Source: CAD feature listing. Evaluate the final solid. Frame: model axes, mm. Face numbers are marked on the shaded views. A direction names the side the tool comes from. Round coordinates to 2 decimals unless told otherwise and drop trailing zeros. Order: outer loops, then holes, each group sorted by start corner. A loop starts at its lowest first (then second) coordinate and runs counter-clockwise, first axis right, second up. Notation, with made-up numbers: (66.25, 71.5) - (99.25, 71.5) arc R29 ccw to (99.25, 101.5) - close; hole circle Ø10 at (-29, -4). An arc over 180 degrees is marked (long way). Return JSON: item names as keys, results as strings. Group by question number.
1) Section A-A, the plane y = 116.5. Give the number of separate pieces and of enclosed holes in the cut face, plus the area to 3 significant figures.
2) Ray query, line 1 (Y direction, x = 128.5, z = -52); line 2 (X direction, y = 83, z = 0); line 3 (Z direction, x = -60, y = 99). Return the intervals inside material, ascending. Write a range as from..to.
3) Section D-D, the plane y = 94. Return loops of the section in (x, z).
4) Section C-C, the plane z = 114.5. Return loops of the section in (x, y).
5) Contact query for flat-ended pins moving along their axis: P1, Ø5.5, axis at x = 30.05, z = -30.05, coming from the +Y side; P2, Ø16, axis at x = -55.5, z = -55.5, coming from the +Y side; P3, Ø5, axis at y = 97.5, z = -16.5, coming from the +X side. Output: stop coordinate, or through.
6) Mould query, pull axis X, two halves, no side actions, for the marked faces 3, 4 and 5. Classes: pulls with the +X half, pulls with the -X half, needs draft (parallel to the pull), parting line crosses it, or undercut.
7) Access query for the marked faces 1 and 2. Directions: +Z, -Z, +X, -X, +Y, -Y. A direction counts if a zero-diameter tool reaches every point of the face in a straight line with its end or side. Return the directions, or none.
8) Section B-B, the plane x = 131. Return loops of the section in (y, z), plus the area to 3 significant figures.
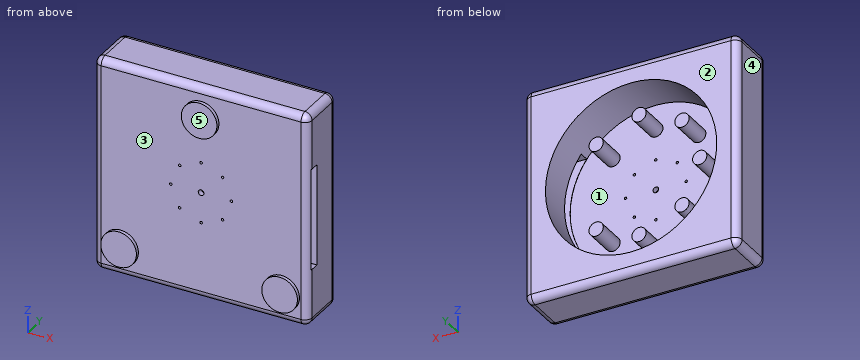
```python
from build123d import *

# Parameters (mm, degrees)
SKETCH_1_W          = 300
SKETCH_1_H          = 300
EXTRUDE_1_DEPTH     = 150
SKETCH_2_R          = 120
CUT_EXTRUDE_1_DEPTH = 62.3
SKETCH_3_R          = 1.75
SKETCH_3_R_2        = 4
CUT_EXTRUDE_2_DEPTH = 10
SKETCH_6_W          = 142.15649329
SKETCH_6_H          = 14
CUT_EXTRUDE_4_DEPTH = 75
SKETCH_11_R         = 10
EXTRUDE_4_DEPTH     = 42.3
FILLET_1_R          = 10
SKETCH_13_W         = 300
SKETCH_13_H         = 300
CUT_EXTRUDE_5_DEPTH = 80
SKETCH_14_R         = 25
EXTRUDE_5_DEPTH     = 5
FILLET_2_R          = 10


with BuildPart() as part:
    # 草图1 → 凸台-拉伸1 (new body)
    with BuildSketch(Plane(origin=(0, 0, 0), x_dir=(1, 0, 0), z_dir=(0, 1, 0))):
        Rectangle(SKETCH_1_W, SKETCH_1_H)
    extrude(amount=EXTRUDE_1_DEPTH)

    # 草图2 → 切除-拉伸1 (cut)
    with BuildSketch(Plane(origin=(0, 150, 0), x_dir=(1, 0, 0), z_dir=(0, 1, 0))):
        with Locations(Location((0, 0, 0), (0, 0, 270))):
            Circle(SKETCH_2_R)
    extrude(amount=-CUT_EXTRUDE_1_DEPTH, mode=Mode.SUBTRACT)

    # 草图3 → 切除-拉伸2 (cut)
    with BuildSketch(Plane(origin=(0, 87.7, 0), x_dir=(1, 0, 0), z_dir=(0, 1, 0))):
        with Locations(Location((42.5, 0, 0), (0, 0, 270))):
            Circle(SKETCH_3_R)
        with Locations(Location((30.0520382, -30.0520382, 0), (0, 0, 270))):
            Circle(SKETCH_3_R)
        with Locations(Location((0, -42.5, 0), (0, 0, 270))):
            Circle(SKETCH_3_R)
        with Locations(Location((-30.0520382, -30.0520382, 0), (0, 0, 270))):
            Circle(SKETCH_3_R)
        with Locations(Location((-42.5, 0, 0), (0, 0, 270))):
            Circle(SKETCH_3_R)
        with Locations(Location((-30.0520382, 30.0520382, 0), (0, 0, 270))):
            Circle(SKETCH_3_R)
        with Locations(Location((0, 42.5, 0), (0, 0, 270))):
            Circle(SKETCH_3_R)
        with Locations(Location((30.0520382, 30.0520382, 0), (0, 0, 270))):
            Circle(SKETCH_3_R)
        with Locations(Location((0, 0, 0), (0, 0, 270))):
            Circle(SKETCH_3_R_2)
    extrude(amount=-CUT_EXTRUDE_2_DEPTH, mode=Mode.SUBTRACT)

    # 草图6 → 切除-拉伸4 (cut)
    with BuildSketch(Plane(origin=(150, 0, 0), x_dir=(0, 0, -1), z_dir=(1, 0, 0))):
        with Locations((0, 95)):
            Rectangle(SKETCH_6_W, SKETCH_6_H)
    extrude(amount=-CUT_EXTRUDE_4_DEPTH, mode=Mode.SUBTRACT)

    # 草图11 → 凸台-拉伸4 (add)
    with BuildSketch(Plane(origin=(0, 87.7, 0), x_dir=(1, 0, 0), z_dir=(0, 1, 0))):
        with Locations(Location((-85, 0, 0), (0, 0, 270))):
            Circle(SKETCH_11_R)
        with Locations(Location((-60.104076401, 60.104076401, 0), (0, 0, 270))):
            Circle(SKETCH_11_R)
        with Locations(Location((0, 85, 0), (0, 0, 270))):
            Circle(SKETCH_11_R)
        with Locations(Location((60.104076401, 60.104076401, 0), (0, 0, 270))):
            Circle(SKETCH_11_R)
        with Locations(Location((60.104076401, -60.104076401, 0), (0, 0, 270))):
            Circle(SKETCH_11_R)
        with Locations(Location((0, -85, 0), (0, 0, 270))):
            Circle(SKETCH_11_R)
        with Locations(Location((-60.104076401, -60.104076401, 0), (0, 0, 270))):
            Circle(SKETCH_11_R)
    extrude(amount=EXTRUDE_4_DEPTH)

    # 圆角1
    fillet_1_edges = [part.edges().sort_by_distance(p)[0] for p in [
        (-150, 150, 0),
        (0, 150, 150),
        (150, 150, 0),
        (0, 0, 150),
        (-150, 0, 0),
        (0, 0, -150),
        (150, 0, 0),
        (150, 75, 150),
        (-150, 75, 150),
        (-150, 75, -150),
        (150, 75, -150),
        (0, 150, -150),
    ]]
    fillet(fillet_1_edges, radius=FILLET_1_R)

    # 草图13 → 切除-拉伸5 (cut)
    with BuildSketch(Plane.XZ):
        Rectangle(SKETCH_13_W, SKETCH_13_H)
    extrude(amount=-CUT_EXTRUDE_5_DEPTH, mode=Mode.SUBTRACT)

    # 草图14 → 凸台-拉伸5 (add)
    with BuildSketch(Plane.XZ.offset(-80)):
        with Locations(Location((0, 104.563725125, 0), (0, 0, 270))):
            Circle(SKETCH_14_R)
        with Locations(Location((-112.815196319, -110.245065947, 0), (0, 0, 270))):
            Circle(SKETCH_14_R)
        with Locations(Location((112.815196319, -110.245065947, 0), (0, 0, 90))):
            Circle(SKETCH_14_R)
    extrude(amount=EXTRUDE_5_DEPTH)

    # 圆角2
    # the kernel refuses this fillet: 10 mm, written as the material it takes off along each edge
    with BuildSketch(Plane(origin=(140, 80, 140), x_dir=(0, 0, 1), z_dir=(-1, 0, 0))) as fillet_2_piece_1:
        with BuildLine():
            CenterArc((10 - FILLET_2_R, FILLET_2_R), FILLET_2_R, 270, 90)
            Line((10, FILLET_2_R), (10, 0))
            Line((10, 0), (10 - FILLET_2_R, 0))
        make_face()
    revolve(axis=Axis((140, 80, 140), (0, 1, 0)), revolution_arc=90, mode=Mode.SUBTRACT)
    with BuildSketch(Plane(origin=(140, 80, -140), x_dir=(1, 0, 0), z_dir=(0, 0, 1))) as fillet_2_piece_2:
        with BuildLine():
            CenterArc((10 - FILLET_2_R, FILLET_2_R), FILLET_2_R, 270, 90)
            Line((10, FILLET_2_R), (10, 0))
            Line((10, 0), (10 - FILLET_2_R, 0))
        make_face()
    revolve(axis=Axis((140, 80, -140), (0, 1, 0)), revolution_arc=90, mode=Mode.SUBTRACT)
    with BuildSketch(Plane(origin=(-140, 80, -140), x_dir=(0, 0, -1), z_dir=(1, 0, 0))) as fillet_2_piece_3:
        with BuildLine():
            CenterArc((10 - FILLET_2_R, FILLET_2_R), FILLET_2_R, 270, 90)
            Line((10, FILLET_2_R), (10, 0))
            Line((10, 0), (10 - FILLET_2_R, 0))
        make_face()
    revolve(axis=Axis((-140, 80, -140), (0, 1, 0)), revolution_arc=90, mode=Mode.SUBTRACT)
    with BuildSketch(Plane(origin=(-140, 80, 140), x_dir=(-1, 0, 0), z_dir=(0, 0, -1))) as fillet_2_piece_4:
        with BuildLine():
            CenterArc((10 - FILLET_2_R, FILLET_2_R), FILLET_2_R, 270, 90)
            Line((10, FILLET_2_R), (10, 0))
            Line((10, 0), (10 - FILLET_2_R, 0))
        make_face()
    revolve(axis=Axis((-140, 80, 140), (0, 1, 0)), revolution_arc=90, mode=Mode.SUBTRACT)
    with BuildSketch(Plane(origin=(-150, 80, -140), x_dir=(1, 0, 0), z_dir=(0, 0, 1)), Plane(origin=(150, 80, 140), x_dir=(-1, 0, 0), z_dir=(0, 0, -1)), Plane(origin=(-140, 80, 150), x_dir=(0, 0, -1), z_dir=(1, 0, 0))) as fillet_2_piece_5:
        with BuildLine():
            CenterArc((FILLET_2_R, FILLET_2_R), FILLET_2_R, 180, 90)
            Line((0, FILLET_2_R), (0, 0))
            Line((0, 0), (FILLET_2_R, 0))
        make_face()
    extrude(amount=280, mode=Mode.SUBTRACT)
    with BuildSketch(Plane(origin=(140, 80, -150), x_dir=(0, 1, 0), z_dir=(-1, 0, 0))) as fillet_2_piece_6:
        with BuildLine():
            CenterArc((FILLET_2_R, -FILLET_2_R), FILLET_2_R, 90, 90)
            Line((0, -FILLET_2_R), (0, 0))
            Line((0, 0), (FILLET_2_R, 0))
        make_face()
    extrude(amount=280, mode=Mode.SUBTRACT)


solid = part.part
```
Geometry check:
{
 "1": {"separate pieces": "8", "enclosed holes": "1", "area": "46,900 mm2"},
 "2": {"line 1": "80..88, 102..150", "line 2": "-147.14..-44.25, -40.75..-4, 4..40.75, 44.25..147.14", "line 3": "-150..-103.92, -70.1..-50.1, 50.1..70.1, 103.92..150"},
 "3": {"outline": "(-150, -140) arc R10 ccw to (-140, -150) - (140, -150) arc R10 ccw to (150, -140) - (150, -71.08) - (96.68, -71.08) arc R120 cw (long way) to (96.68, 71.08) - (150, 71.08) - (150, 140) arc R10 ccw to (140, 150) - (-140, 150) arc R10 ccw to (-150, 140) - close; circle Ø20 at (-85, 0); circle Ø20 at (-60.1, -60.1); circle Ø20 at (-60.1, 60.1); circle Ø20 at (0, -85); circle Ø20 at (0, 85); circle Ø20 at (60.1, -60.1); circle Ø20 at (60.1, 60.1)"},
 "4": {"outline": "(-150, 90) arc R10 ccw to (-140, 80) - (-22.94, 80) - (-22.94, 75) - (22.94, 75) - (22.94, 80) - (140, 80) arc R10 ccw to (150, 90) - (150, 140) arc R10 ccw to (140, 150) - (35.91, 150) - (35.91, 87.7) - (-35.91, 87.7) - (-35.91, 150) - (-140, 150) arc R10 ccw to (-150, 140) - close"},
 "5": {"P1": "y = 87.7", "P2": "y = 130", "P3": "x = -118.49"},
 "6": {"face 3": "undercut", "face 4": "pulls with the -X half", "face 5": "needs draft"},
 "7": {"face 1": "+Y", "face 2": "+Z, -Z, +X, -X, +Y"},
 "8": {"outline": "(75, -127.4) - (80, -127.4) - (80, -140) arc R10 ccw to (90, -150) - (140, -150) arc R10 ccw to (150, -140) - (150, 140) arc R10 ccw to (140, 150) - (90, 150) arc R10 ccw to (80, 140) - (80, -93.09) - (75, -93.09) - close; hole (88, -71.08) - (102, -71.08) - (102, 71.08) - (88, 71.08) - close", "area": "19,100 mm2"}
}
